Build history of the part. All positions in model axes, mm. A direction names the side the tool comes from. Round coordinates to 2 decimals unless told otherwise and drop trailing zeros. Loops run counter-clockwise (first coordinate to the right, second up) from the corner with the lowest first, then second, coordinate; pieces in that order, holes last. Notation, with made-up numbers: (66.5, 78.5) -> (74.5, 78.5) arc R32 cw to (74.5, 108.5) -> close; hole circle Ø10 at (38.5, 7). An arc over 180 degrees is marked (long way). Put each result on its own line as item: value. Start each with the question number.
Item 1: Tool access for faces 4 (the flat face through (-69.85, 3, 0)), 5 (the flat face through (-35, 9, -7)), 6 (the cylindrical face through (31.765, 6.972, -34.641)): list every direction of +Z, -Z, +X, -X, +Y, -Y with a clear straight run to the whole face (end or side of a thin tool).
Item 2: Cut at A-A, the plane y = 6.5. List the corners of the cut face in (x, z), plus the area to 3 significant figures.
Item 3: Flat gauge pin, fed straight in: pin 1 Ø2 at (x, z) = (91, 55) entering from +Y. Where does the tip first touch, or does it go through?
Item 4: Cut at B-B, the plane z = -7. List the corners of the cut face in (x, y).
Item 5: Pull direction X, two halves, no side cores. Call faces 1 (the flat face through (120, 2, 24)), 2 (the cylindrical face through (-21, 4, -28)), 3 (the flat face through (25, 5, 43)): +X half, -X half, draft (parallel to the pull), parting line (faces both ways), or undercut.
Item 6: Cut at C-C, the plane x = 28.5. List the corners of the cut face in (y, z).
Item 7: Cut at D-D, the plane x = 57. List the corners of the cut face in (y, z).
Item 8: Drill centre lines: probe 1 along X at (y, z) = (4.25, -41); probe 2 along Z at (x, y) = (41, 4); probe 3 along X at (y, z) = (0.5, -6.5). Where is each one in solid material? Low to high. Write a range as [from, to].
```python
from build123d import *

# Parameters (mm, degrees)
SCHIZZO1_W                   = 240
SCHIZZO1_H                   = 195
SCHIZZO1_R                   = 35
ESTRUSIONE_ESTRUSIONE1_DEPTH = 5
SCHIZZO3_R                   = 47
SCHIZZO3_R_2                 = 35
ESTRUSIONE_ESTRUSIONE2_DEPTH = 4
FORO_PER_VITE_M3_1_D         = 4.5
FORO_PER_VITE_M3_1_DEPTH     = 18.1
FORO_PER_VITE_M3_1_TIP       = 1.351936393
SCHIZZO7_W                   = 42.3
SCHIZZO7_H                   = 42.3
TAGLIO_ESTRUSIONE1_DEPTH     = 14


with BuildPart() as part:
    # Schizzo1 → Estrusione-Estrusione1 (new body)
    with BuildSketch(Plane(origin=(0, 0, 0), x_dir=(1, 0, 0), z_dir=(0, 1, 0))):
        with Locations((0, -22.5)):
            Rectangle(SCHIZZO1_W, SCHIZZO1_H)
        with Locations(Location((0, 0, 0), (0, 0, 270))):
            Circle(SCHIZZO1_R, mode=Mode.SUBTRACT)
    extrude(amount=ESTRUSIONE_ESTRUSIONE1_DEPTH)

    # Schizzo3 → Estrusione-Estrusione2 (add)
    with BuildSketch(Plane(origin=(0, 5, 0), x_dir=(1, 0, 0), z_dir=(0, 1, 0))):
        with Locations(Location((0, 0, 0), (0, 0, 270))):
            Circle(SCHIZZO3_R)
        with Locations(Location((0, 0, 0), (0, 0, 270))):
            Circle(SCHIZZO3_R_2, mode=Mode.SUBTRACT)
    extrude(amount=ESTRUSIONE_ESTRUSIONE2_DEPTH)

    # Foro per Vite M3-1
    with Locations(Plane(origin=(0, 0, 0), x_dir=(-1, 0, 0), z_dir=(0, -1, 0))):
        with Locations((-41, 0), (0, 41), (41, 0), (0, -41)):
            Hole(FORO_PER_VITE_M3_1_D / 2, depth=FORO_PER_VITE_M3_1_DEPTH)
            with Locations((0, 0, -(FORO_PER_VITE_M3_1_DEPTH + FORO_PER_VITE_M3_1_TIP / 2))):  # 118° drill point
                Cone(0, FORO_PER_VITE_M3_1_D / 2, FORO_PER_VITE_M3_1_TIP, mode=Mode.SUBTRACT)

    # Schizzo7 → Taglio-Estrusione1 (cut)
    with BuildSketch(Plane(origin=(0, 5, 0), x_dir=(1, 0, 0), z_dir=(0, 1, 0))):
        with Locations((-91, 0)):
            Rectangle(SCHIZZO7_W, SCHIZZO7_H)
    extrude(amount=-TAGLIO_ESTRUSIONE1_DEPTH, mode=Mode.SUBTRACT)


solid = part.part
```
Reply:
1. face 4: +Y, -Y
1. face 5: +Z, -Z, +X, -X, +Y
1. face 6: +Y
2. outline: circle Ø94 at (0, 0); hole circle Ø4.5 at (-41, 0); hole circle Ø70 at (0, 0); hole circle Ø4.5 at (0, -41); hole circle Ø4.5 at (0, 41); hole circle Ø4.5 at (41, 0)
2. area: 3,030 mm^2
3. pin 1: stops at y = 5
4. outline: (-120, 0) -> (-112.15, 0) -> (-112.15, 5) -> (-120, 5) -> close; (-69.85, 0) -> (-34.29, 0) -> (-34.29, 9) -> (-46.48, 9) -> (-46.48, 5) -> (-69.85, 5) -> close; (34.29, 0) -> (120, 0) -> (120, 5) -> (46.48, 5) -> (46.48, 9) -> (34.29, 9) -> close
5. face 1: +X half
5. face 2: undercut
5. face 3: draft
6. outline: (0, -75) -> (5, -75) -> (5, -37.37) -> (9, -37.37) -> (9, -20.32) -> (0, -20.32) -> close; (0, 20.32) -> (9, 20.32) -> (9, 37.37) -> (5, 37.37) -> (5, 120) -> (0, 120) -> close
7. outline: (0, -75) -> (5, -75) -> (5, 120) -> (0, 120) -> close
8. probe 1: x = [-120, -2.25], [2.25, 120]
8. probe 2: z = [-75, -2.25], [2.25, 120]
8. probe 3: x = [-120, -112.15], [-69.85, -34.39], [34.39, 120]
